Check sheet for the drawn part. Datum: minimum x, y, z corner. Units: mm. A direction names the side the tool comes from. Give positions to 0.01 mm unless a question says otherwise; leave off trailing zeros. Write each loop counter-clockwise with the first axis right and the second up, starting at its lowest first coordinate (ties: lowest second). Pieces come first, ordered by that corner, then holes. Notation, with made-up numbers: M 13,30.25 L 29,30.25 A17 cw 29,57.25 Z; hole C 57,-11.5 d1. An arc over 180 degrees is marked long. Use CSV: the item, a comma, the result in double quotes. Start each with the question number.
1. Cross-section at A-A, the plane x = 45. Enter the section's corners in (y, z).
2. Cross-section at B-B, the plane y = 45. Enter the section's corners in (x, z).
3. Cross-section at C-C, the plane y = 24.5. Enter the section's corners in (x, z).
4. Depth check by flat-ended pin: P1, Ø12, axis at x = 20.5, y = 44, coming from the -Z side; P2, Ø2, axis at x = 58.5, z = 207.5, coming from the -Y side; P3, Ø10, axis at x = 65, z = 187.5, coming from the -Y side (1 decimal); P4, Ø4, axis at x = 81.77, y = 8.23, coming from the +Z side. Enter the tip coordinate at first touch or a pass-through.
5. Cross-section at D-D, the plane y = 63. Enter the section's corners in (x, z).
6. Scan lines: line 1 (Y direction, x = 81.5, z = 96) (1 decimal); line 2 (Z direction, x = 45, y = 37.5); line 3 (Z direction, x = 18, y = 8). Record each from-to range of solid material in increasing order.
7. Access from +Z, -Z, +X, -X, +Y, -Y to the whole of each face (thin tool, end or side, straight path). Record for the marked faces 1, 2 and 3.
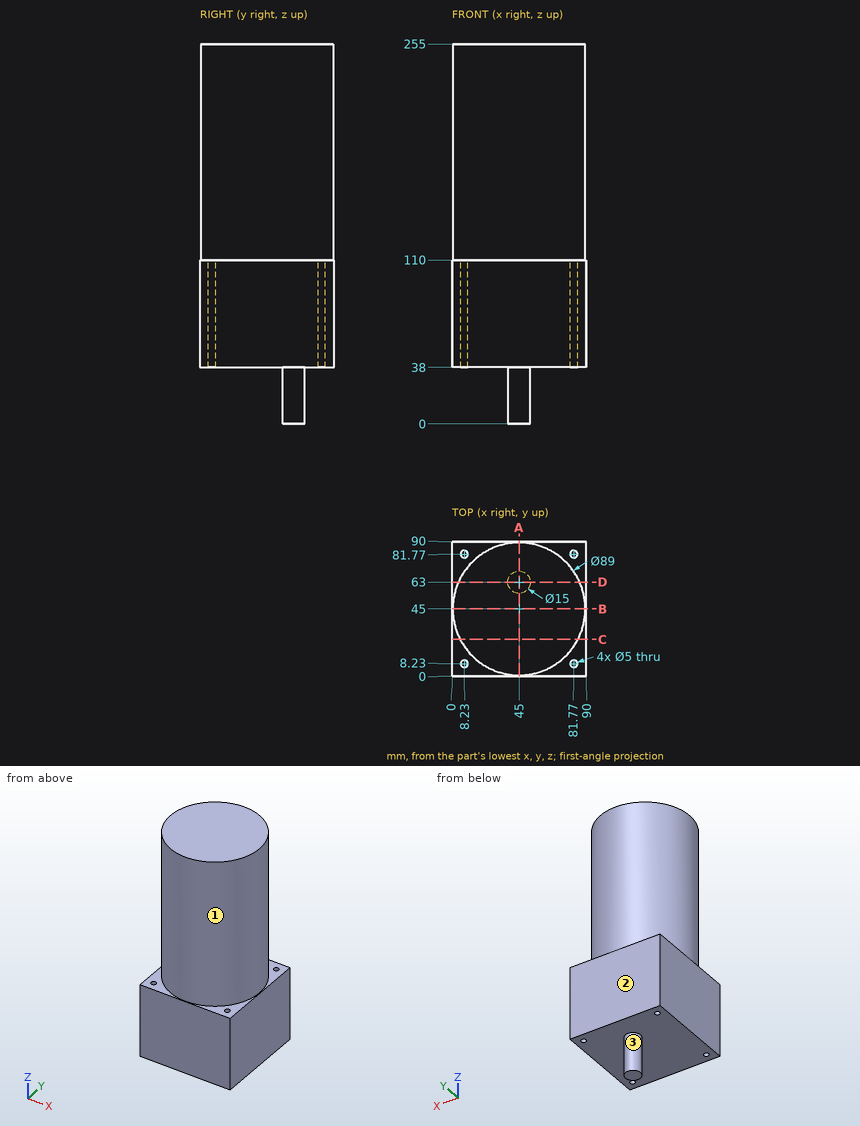
Worked answers:
1,outline,"M 0,38 L 55.5,38 L 55.5,0 L 70.5,0 L 70.5,38 L 90,38 L 90,110 L 89.5,110 L 89.5,255 L 0.5,255 L 0.5,110 L 0,110 Z"
2,outline,"M 0,38 L 90,38 L 90,110 L 89.5,110 L 89.5,255 L 0.5,255 L 0.5,110 L 0,110 Z"
3,outline,"M 0,38 L 90,38 L 90,110 L 84.5,110 L 84.5,255 L 5.5,255 L 5.5,110 L 0,110 Z"
4,P1,"stops at z = 38"
4,P2,"stops at y = 2.29"
4,P3,"stops at y = 3.1"
4,P4,"passes through"
5,outline,"M 0,38 L 37.5,38 L 37.5,0 L 52.5,0 L 52.5,38 L 90,38 L 90,110 L 85.7,110 L 85.7,255 L 4.3,255 L 4.3,110 L 0,110 Z"
6,line 1,"y = 0 to 5.7, 10.7 to 79.3, 84.3 to 90"
6,line 2,"z = 38 to 255"
6,line 3,"z = 38 to 110"
7,face 1,"+Z"
7,face 2,"+Z, -Z, +X, -X, +Y"
7,face 3,"-Z"
